Design review of the part built by this model. Coordinates are the model's own, in mm. Coordinates: 2 decimals unless noted, no trailing zeros. Write each loop counter-clockwise with the first axis right and the second up, starting at its lowest first coordinate (ties: lowest second). Pieces come first, ordered by that corner, then holes. Notation, with made-up numbers: (77.5, 1) - (101.5, 1) arc R16 ccw to (101.5, 22) - close; hole circle Ø3 at (34, 1.5). An arc over 180 degrees is marked (long way). Use a Markdown table: item, result.
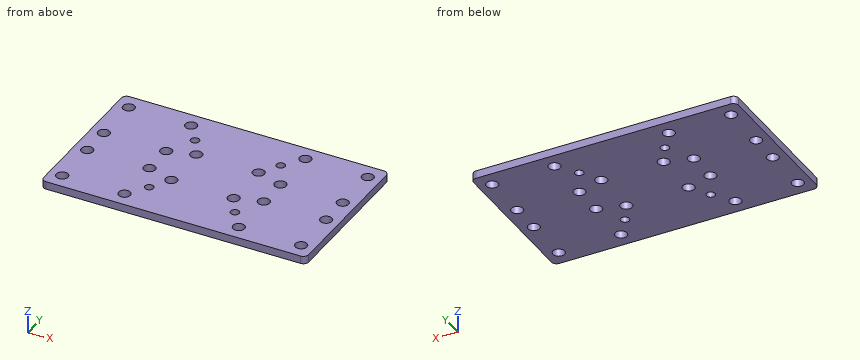
Autodesk Inventor part; units mm, degrees
ref_plane "YZ Plane" through (0, 0, 0) normal (1, 0, 0) x (0, 1, 0)
ref_plane "XZ Plane" through (0, 0, 0) normal (0, 1, 0) x (-1, 0, 0)
ref_plane "XY Plane" through (0, 0, 0) normal (0, 0, 1) x (1, 0, 0)
sketch "Sketch1" plane through (0, 0, 0) normal (0, 0, 1) x (1, 0, 0)
  line L0 (-51, -30) -> (51, -30)
  line L1 (51, -30) -> (51, 30)
  line L2 (51, 30) -> (-51, 30)
  line L3 (-51, 30) -> (-51, -30)
  line L4 (-51, -30) -> (51, 30) construction
  line L5 (51, -30) -> (-51, 30) construction
  point P0 (0, 0)
  dimension "d0" = 102
  dimension "d3" = 60
extrude "Extrusion1" add sketch "Sketch1" along normal blind 3
sketch "Sketch2" plane through (0, 0, 3) normal (0, 0, 1) x (1, 0, 0)
  line L0 (22, -24) -> (46, -24)
  line L1 (46, -24) -> (46, -6)
  line L2 (46, -6) -> (22, -6)
  line L3 (22, -6) -> (22, -24)
  line L4 (22, -24) -> (46, -6) construction
  line L5 (46, -24) -> (22, -6) construction
  line L6 (-51, -30) -> (51, -30)
  line L7 (51, -30) -> (51, 30)
  circle A0 centre (46, -6) radius 2.25
  circle A1 centre (46, -24) radius 2.25
  circle A2 centre (22, -24) radius 2.25
  circle A3 centre (22, -6) radius 2.25
  point P0 (0, 0)
  point P1 (34, -15)
  dimension "d4" = 24
  dimension "d5" = 18
  dimension "d6" = 15
  dimension "d7" = 5
  dimension "d8" = 4.5
  dimension "d9" = 4.5
  dimension "d10" = 4.5
  dimension "d11" = 4.5
extrude "Extrusion2" cut sketch "Sketch2" against normal blind 3 contours L3 A2 L0 | L0 A2 L3 | A1 L1 L0 | L0 L1 A1 | A3 L2 L3 | L3 L2 A3 | A0 L2 L1 | L1 L2 A0
pattern_linear "Rectangular Pattern1" count 2 spacing 30 along (0, 1, 0) of "Extrusion2"
sketch "Sketch3" plane through (0, 0, 3) normal (0, 0, 1) x (1, 0, 0)
  line L0 (-12, -9) -> (12, -9)
  line L1 (12, -9) -> (12, 9)
  line L2 (12, 9) -> (-12, 9)
  line L3 (-12, 9) -> (-12, -9)
  line L4 (-12, -9) -> (12, 9) construction
  line L5 (12, -9) -> (-12, 9) construction
  circle A0 centre (-12, 9) radius 2.25
  circle A1 centre (12, 9) radius 2.25
  circle A2 centre (12, -9) radius 2.25
  circle A3 centre (-12, -9) radius 2.25
  point P0 (0, 0)
  dimension "d20" = 24
  dimension "d21" = 18
  dimension "d22" = 4.5
  dimension "d23" = 4.5
  dimension "d24" = 4.5
  dimension "d25" = 4.5
extrude "Extrusion3" cut sketch "Sketch3" against normal blind 3 contours L3 A3 L0 | L0 A3 L3 | A2 L1 L0 | L0 L1 A2 | A0 L2 L3 | L3 L2 A0 | A1 L2 L1 | L1 L2 A1
sketch "Sketch4" plane through (0, 0, 3) normal (0, 0, 1) x (1, 0, 0)
  line L0 (-16.5, -16.5) -> (16.5, -16.5)
  line L1 (16.5, -16.5) -> (16.5, 16.5)
  line L2 (16.5, 16.5) -> (-16.5, 16.5)
  line L3 (-16.5, 16.5) -> (-16.5, -16.5)
  line L4 (-16.5, -16.5) -> (16.5, 16.5) construction
  line L5 (16.5, -16.5) -> (-16.5, 16.5) construction
  circle A0 centre (16.5, 16.5) radius 1.65
  circle A1 centre (-16.5, 16.5) radius 1.65
  circle A2 centre (-16.5, -16.5) radius 1.65
  circle A3 centre (16.5, -16.5) radius 1.65
  point P0 (0, 0)
  dimension "d28" = 33
  dimension "d29" = 33
  dimension "d30" = 3.3
  dimension "d31" = 3.3
  dimension "d32" = 3.3
  dimension "d33" = 3.3
extrude "Extrusion4" cut sketch "Sketch4" against normal blind 3 contours L3 A2 L0 | L0 A2 L3 | A3 L1 L0 | L0 L1 A3 | A1 L2 L3 | L3 L2 A1 | A0 L2 L1 | L1 L2 A0
mirror "Mirror1" about plane through (0, 0, 0) normal (1, 0, 0) of "Extrusion2", "Rectangular Pattern1"
fillet "Fillet1" radius 2 4 edges at (51, 30, 1.5) (51, -30, 1.5) (-51, -30, 1.5) (-51, 30, 1.5)
properties part number "De truc Z"
(1) Take a section at B-B on z = 0.55. State how many separate pieces and enclosed holes the cut face has, and give its area (3 significant figures).
Determined:
| item | result |
|---|---|
| separate pieces | 1 |
| enclosed holes | 24 |
| area | 5,760 mm2 |
(2) Take a section at D-D on y = -25. Write out the cut boundary in (x, z).
Determined:
| item | result |
|---|---|
| outline | (-51, 0) - (-48.02, 0) - (-48.02, 3) - (-51, 3) - close; (-43.98, 0) - (-24.02, 0) - (-24.02, 3) - (-43.98, 3) - close; (-19.98, 0) - (19.98, 0) - (19.98, 3) - (-19.98, 3) - close; (24.02, 0) - (43.98, 0) - (43.98, 3) - (24.02, 3) - close; (48.02, 0) - (51, 0) - (51, 3) - (48.02, 3) - close |
(3) For L1, parallel to X at y = -24, z = 1.5; L2, parallel to Y at x = -46, z = 2.15; L3, parallel to X at y = 16.5, z = 2.1, list the stretches that pass through material, from the lowest coordinate up. Write a range as from..to.
Determined:
| item | result |
|---|---|
| L1 | -51..-48.25, -43.75..-24.25, -19.75..19.75, 24.25..43.75, 48.25..51 |
| L2 | -30..-26.25, -21.75..-8.25, -3.75..3.75, 8.25..21.75, 26.25..30 |
| L3 | -51..-18.15, -14.85..14.85, 18.15..51 |
(4) Take a section at C-C on x = 46. Write out the cut boundary in (y, z).
Determined:
| item | result |
|---|---|
| outline | (-30, 0) - (-26.25, 0) - (-26.25, 3) - (-30, 3) - close; (-21.75, 0) - (-8.25, 0) - (-8.25, 3) - (-21.75, 3) - close; (-3.75, 0) - (3.75, 0) - (3.75, 3) - (-3.75, 3) - close; (8.25, 0) - (21.75, 0) - (21.75, 3) - (8.25, 3) - close; (26.25, 0) - (30, 0) - (30, 3) - (26.25, 3) - close |
(5) Take a section at A-A on x = 16.5. Write out the cut boundary in (y, z).
Determined:
| item | result |
|---|---|
| outline | (-30, 0) - (-18.15, 0) - (-18.15, 3) - (-30, 3) - close; (-14.85, 0) - (14.85, 0) - (14.85, 3) - (-14.85, 3) - close; (18.15, 0) - (30, 0) - (30, 3) - (18.15, 3) - close |
(6) For pin 1 (3.5 mm diameter, centred on x = -46, y = 24, fed in from +Z), flat-tipped, find the tip position at first contact; note if it passes through.
Determined:
| item | result |
|---|---|
| pin 1 | through |
